The model under review builds one solid part; all positions refer to its coordinate system, in mm. Face numbers are marked on the shaded views. A direction names the side the tool comes from. Give positions to 0.01 mm unless a question says otherwise; leave off trailing zeros. Loops run counter-clockwise (first coordinate to the right, second up) from the corner with the lowest first, then second, coordinate; pieces in that order, holes last. Notation, with made-up numbers: M 9,37 L 31,37 A27 ccw 31,54 Z; hole C 59.5,54.25 d2. An arc over 180 degrees is marked long. Write item = value, one per line. Start each with the question number.
1. We need section B-B on x = 0. Count the separate pieces of the cut face and the enclosed holes in it, then the cut area to 3 significant figures.
2. For the marked faces 4, 5, 6, 7 and 8, list the 3-axis set-ups (+Z, -Z, +X, -X, +Y, -Y) from which the entire face can be reached by the end or side of a thin tool; tool diameter is ignored.
3. We need section A-A on y = 9.5. Give the boundary of the cut face in (x, z).
4. For pin 1 (12 mm diameter, centred on x = 6, y = 18, fed in from -Z); pin 2 (1 mm diameter, centred on x = -17.5, y = -8.5, fed in from +Z); pin 3 (3 mm diameter, centred on y = 16, z = 19.5, fed in from -X), all flat-tipped, find the tip position at first contact; note any pin that passes through.
5. Draft analysis for pull direction Y (two halves, no side actions). For the marked faces 1, 2 and 3, state which applies: pulls with the +Y half, pulls with the -Y half, needs draft (parallel to the pull), parting line crosses it, or undercut.
6. We need section D-D on x = -24. Give the boundary of the cut face in (y, z).
7. Wall thickness on line 1 along Y through (x, z) = (0, -12.25); line 2 along Y through (x, z) = (27, -8); line 3 along X through (y, z) = (-28, 12.5): over which ranges is each line inside the solid? List them lowest first. Write a range as from..to.
from build123d import *

# Parameters (mm, degrees)
CUT_EXTRUDE1_DEPTH      = 57.315677826
CUT_EXTRUDE1_DEPTH_BACK = 57.315677826
SKETCH2_W               = 52
SKETCH2_H               = 45
FILLET1_R               = 8
BOSS_EXTRUDE1_DEPTH     = 56
CUT_EXTRUDE2_DEPTH      = 62.715224497
CUT_EXTRUDE2_DEPTH_BACK = 62.715224497
SKETCH4_R               = 8
FILLET2_START           = -17
FILLET2_DEPTH           = 34
CUT_EXTRUDE3_DEPTH      = 0.4


with BuildPart() as part:
    # Sketch1 → Revolve1 (revolve)
    with BuildSketch(Plane.XY):
        Polygon((0, 35.952879581), (-30.5, 35.952879581), (-30.5, 24.792879581), (-26.5, 24.792879581), (-26.5, 22.792879581), (-30.5, 22.792879581), (-30.5, 15.792879581), (-26.5, 15.792879581), (-26.5, 13.792879581), (-30.5, 13.792879581), (-30.5, 3.792879581), (-26.5, 3.792879581), (-26.5, 0.792879581), (-30.5, 0.792879581), (-30.5, -36.207120419), (-17.7, -36.207120419), (-17.7, 22.952879581), (0, 22.952879581), align=None)
    revolve(axis=Axis((0, 39.251308901, 0), (0, -1, 0)))

    # Sketch2 → Cut-Extrude1 (cut, two sides: drawn at the far end of the back side and taken through both)
    with BuildSketch(Plane.XY.offset(-CUT_EXTRUDE1_DEPTH_BACK)):
        with Locations((0, -36.207120419)):
            Rectangle(SKETCH2_W, SKETCH2_H)
    extrude(amount=CUT_EXTRUDE1_DEPTH + CUT_EXTRUDE1_DEPTH_BACK, mode=Mode.SUBTRACT)

    # Fillet1
    fillet1_edges = [part.edges().sort_by_distance(p)[0] for p in [
        (26, -13.707120419, 0),
        (-26, -13.707120419, 0),
    ]]
    fillet(fillet1_edges, radius=FILLET1_R)

    # Sketch3 → Boss-Extrude1 (add)
    with BuildSketch(Plane.XZ.offset(-22.952879581)):
        with BuildLine():
            Line((-15.186081342, -9.092465753), (15.186081342, -9.092465753))
            ThreePointArc((15.186081342, -9.092465753), (0, -17.7), (-15.186081342, -9.092465753))
        make_face()
        with BuildLine():
            Line((-15.186081342, 9.092465753), (15.186081342, 9.092465753))
            ThreePointArc((15.186081342, 9.092465753), (0, 17.7), (-15.186081342, 9.092465753))
        make_face()
    extrude(amount=BOSS_EXTRUDE1_DEPTH)

    # Sketch4 → Cut-Extrude2 (cut, two sides: drawn at the far end of the back side and taken through both)
    with BuildSketch(Plane.XY.offset(-9.092465753).offset(-CUT_EXTRUDE2_DEPTH_BACK)):
        with Locations((0, -23.707120419)):
            Circle(SKETCH4_R)
    extrude(amount=CUT_EXTRUDE2_DEPTH + CUT_EXTRUDE2_DEPTH_BACK, mode=Mode.SUBTRACT)

    # Fillet2: read off the stored shape, not the designer's step
    # Fillet2 outline → Fillet2 (cut)
    with BuildSketch(Plane.XY.offset(FILLET2_START)):
        with BuildLine():
            Line((30.749452468, -36.207120419), (30.500160015, -36.182073684))
            ThreePointArc((30.500160015, -36.182073684), (27.291954698, -34.561282019), (26, -31.207120419))
            Line((26, -31.207120419), (26, -36.207120419))
            Line((26, -36.207120419), (30.749452468, -36.207120419))
        make_face()
        with BuildLine():
            Line((-26, -36.207120419), (-26, -31.207120419))
            ThreePointArc((-26, -31.207120419), (-27.291900757, -34.561222386), (-30.500000003, -36.182057605))
            Line((-30.500000003, -36.182057605), (-30.749371855, -36.207120419))
            Line((-30.749371855, -36.207120419), (-26, -36.207120419))
        make_face()
    extrude(amount=FILLET2_DEPTH, mode=Mode.SUBTRACT)

    # Sketch5 → Cut-Extrude3 (cut)
    with BuildSketch(Plane(origin=(0, 35.952879581, 0), x_dir=(1, 0, 0), z_dir=(0, 1, 0))):
        with BuildLine():
            Line((-8.5, -11.466567669), (8.5, -11.466567669))
            ThreePointArc((8.5, -11.466567669), (16.696900168, -3.232277046), (9.94436139, 6.222665285))
            ThreePointArc((9.94436139, 6.222665285), (0, 17.276077147), (-9.94436139, 6.222665285))
            ThreePointArc((-9.94436139, 6.222665285), (-16.696900168, -3.232277046), (-8.5, -11.466567669))
        make_face()
    extrude(amount=-CUT_EXTRUDE3_DEPTH, mode=Mode.SUBTRACT)


solid = part.part
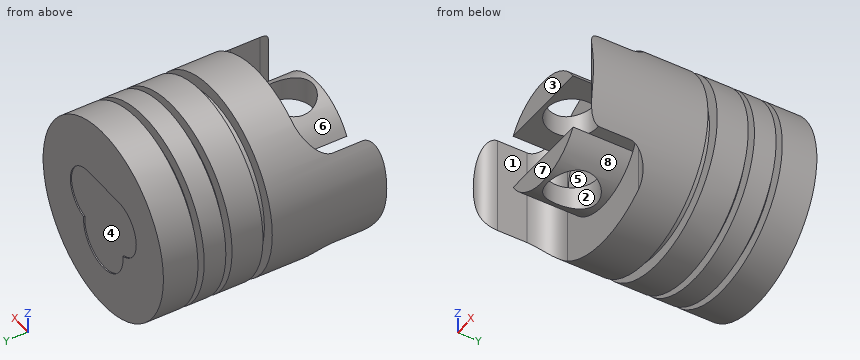
Final values:
q1.separate_pieces = 3
q1.enclosed_holes = 0
q1.area = 2,350 mm²
q2.face_4 = +Y
q2.face_5 = -Y
q2.face_6 = +Z, -Y
q2.face_7 = +Z, -Z, -Y
q2.face_8 = -Z, -Y
q3.outline = C 0,0 d61; hole M -15.19,-9.09 L 15.19,-9.09 A17.7 ccw 15.19,9.09 L -15.19,9.09 A17.7 ccw Z
q4.pin_1 = -30.5
q4.pin_2 = 25.32
q4.pin_3 = -24.62
q5.face_1 = needs draft
q5.face_2 = undercut
q5.face_3 = pulls with the -Y half
q6.outline = M -16.42,-18.82 L 0.79,-18.82 L 0.79,-11.24 L 3.79,-11.24 L 3.79,-18.82 L 13.79,-18.82 L 13.79,-11.24 L 15.79,-11.24 L 15.79,-18.82 L 22.79,-18.82 L 22.79,-11.24 L 24.79,-11.24 L 24.79,-18.82 L 35.95,-18.82 L 35.95,18.82 L 24.79,18.82 L 24.79,11.24 L 22.79,11.24 L 22.79,18.82 L 15.79,18.82 L 15.79,11.24 L 13.79,11.24 L 13.79,18.82 L 3.79,18.82 L 3.79,11.24 L 0.79,11.24 L 0.79,18.82 L -16.42,18.82 Z
q7.line_1 = -33.05..-31.71, -15.71..35.55
q7.line_2 = -34.21..0.79, 3.79..13.79, 15.79..22.79, 24.79..35.95
q7.line_3 = -27.82..-26, -12.53..-6.75, 6.75..12.53, 26..27.82
